The model under review builds one solid part; all positions refer to its coordinate system, in mm. Face numbers are marked on the shaded views. Give positions to 0.01 mm unless a question says otherwise; leave off trailing zeros. Loops run counter-clockwise (first coordinate to the right, second up) from the corner with the lowest first, then second, coordinate; pieces in that order, holes last. Notation, with made-up numbers: M -12.5,62.5 L 14.5,62.5 A21 ccw 14.5,96.5 Z; hole C 66.5,5.25 d4. An arc over 180 degrees is marked long. Return JSON: item names as keys, results as strings. Group by question number.
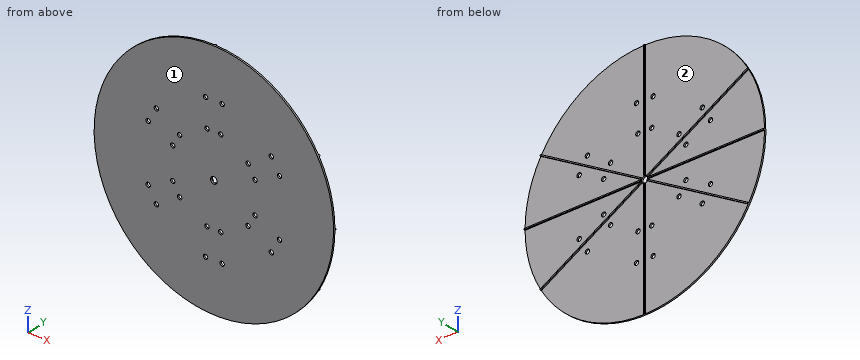
```python
from build123d import *

# Parameters (mm, degrees)
SKETCH1_R           = 217.5
SKETCH1_R_2         = 4
SKETCH1_R_3         = 6
BOSS_EXTRUDE1_DEPTH = 2.5
CUT_EXTRUDE1_START  = -2
SKETCH2_R           = 4
SKETCH2_R_2         = 6
CUT_EXTRUDE1_DEPTH  = 2


with BuildPart() as part:
    # Sketch1 → Boss-Extrude1 (new, symmetric)
    with BuildSketch(Plane(origin=(0, 0, 0), x_dir=(1, 0, 0), z_dir=(0, 1, 0))):
        with Locations(Location((0, 0, 0), (0, 0, 270))):
            Circle(SKETCH1_R)
        with Locations(Location((-12.5, 79.017403146, 0), (0, 0, 270))):
            Circle(SKETCH1_R_2, mode=Mode.SUBTRACT)
        with Locations(Location((12.5, 79.017403146, 0), (0, 0, 270))):
            Circle(SKETCH1_R_2, mode=Mode.SUBTRACT)
        with Locations(Location((62.181078466, 50.334019121, 0), (0, 0, 270))):
            Circle(SKETCH1_R_2, mode=Mode.SUBTRACT)
        with Locations(Location((74.681078466, 28.683384026, 0), (0, 0, 270))):
            Circle(SKETCH1_R_2, mode=Mode.SUBTRACT)
        with Locations(Location((74.681078466, -28.683384026, 0), (0, 0, 270))):
            Circle(SKETCH1_R_2, mode=Mode.SUBTRACT)
        with Locations(Location((62.181078466, -50.334019121, 0), (0, 0, 270))):
            Circle(SKETCH1_R_2, mode=Mode.SUBTRACT)
        with Locations(Location((12.5, -79.017403146, 0), (0, 0, 270))):
            Circle(SKETCH1_R_2, mode=Mode.SUBTRACT)
        with Locations(Location((-12.5, -79.017403146, 0), (0, 0, 270))):
            Circle(SKETCH1_R_2, mode=Mode.SUBTRACT)
        with Locations(Location((-62.181078466, -50.334019121, 0), (0, 0, 270))):
            Circle(SKETCH1_R_2, mode=Mode.SUBTRACT)
        with Locations(Location((-74.681078466, -28.683384026, 0), (0, 0, 270))):
            Circle(SKETCH1_R_2, mode=Mode.SUBTRACT)
        with Locations(Location((-74.681078466, 28.683384026, 0), (0, 0, 270))):
            Circle(SKETCH1_R_2, mode=Mode.SUBTRACT)
        with Locations(Location((-62.181078466, 50.334019121, 0), (0, 0, 270))):
            Circle(SKETCH1_R_2, mode=Mode.SUBTRACT)
        with Locations(Location((15, 129.131715701, 0), (0, 0, 270))):
            Circle(SKETCH1_R_2, mode=Mode.SUBTRACT)
        with Locations(Location((-15, 129.131715701, 0), (0, 0, 90))):
            Circle(SKETCH1_R_2, mode=Mode.SUBTRACT)
        with Locations(Location((104.331346232, 77.556238907, 0), (0, 0, 90))):
            Circle(SKETCH1_R_2, mode=Mode.SUBTRACT)
        with Locations(Location((119.331346232, 51.575476794, 0), (0, 0, 270))):
            Circle(SKETCH1_R_2, mode=Mode.SUBTRACT)
        with Locations(Location((119.331346232, -51.575476794, 0), (0, 0, 90))):
            Circle(SKETCH1_R_2, mode=Mode.SUBTRACT)
        with Locations(Location((104.331346232, -77.556238907, 0), (0, 0, 270))):
            Circle(SKETCH1_R_2, mode=Mode.SUBTRACT)
        with Locations(Location((15, -129.131715701, 0), (0, 0, 90))):
            Circle(SKETCH1_R_2, mode=Mode.SUBTRACT)
        with Locations(Location((-15, -129.131715701, 0), (0, 0, 270))):
            Circle(SKETCH1_R_2, mode=Mode.SUBTRACT)
        with Locations(Location((-104.331346232, -77.556238907, 0), (0, 0, 90))):
            Circle(SKETCH1_R_2, mode=Mode.SUBTRACT)
        with Locations(Location((-119.331346232, -51.575476794, 0), (0, 0, 270))):
            Circle(SKETCH1_R_2, mode=Mode.SUBTRACT)
        with Locations(Location((-119.331346232, 51.575476794, 0), (0, 0, 90))):
            Circle(SKETCH1_R_2, mode=Mode.SUBTRACT)
        with Locations(Location((-104.331346232, 77.556238907, 0), (0, 0, 270))):
            Circle(SKETCH1_R_2, mode=Mode.SUBTRACT)
        with Locations(Location((0, 0, 0), (0, 0, 270))):
            Circle(SKETCH1_R_3, mode=Mode.SUBTRACT)
    extrude(amount=BOSS_EXTRUDE1_DEPTH, both=True)

    # Sketch2 → Cut-Extrude1 (cut)
    with BuildSketch(Plane(origin=(0, 2.5, 0), x_dir=(1, 0, 0), z_dir=(0, 1, 0)).offset(CUT_EXTRUDE1_START)):
        with BuildLine():
            ThreePointArc((-217.497701137, -1), (-210.088867218, -56.29314231), (-188.85853445, -107.882825165))
            Line((-188.85853445, -107.882825165), (-5.888022785, -2.244751001))
            ThreePointArc((-5.888022785, -2.244751001), (-5.457177799, -3.150703071), (-4.888022785, -3.976801809))
            Line((-4.888022785, -3.976801809), (-187.85853445, -109.614875972))
            ThreePointArc((-187.85853445, -109.614875972), (-108.75, -188.360525323), (-1, -217.497701137))
            Line((-1, -217.497701137), (-1, -6.22155281))
            ThreePointArc((-1, -6.22155281), (0, -6.301406142), (1, -6.22155281))
            Line((1, -6.22155281), (1, -217.497701137))
            ThreePointArc((1, -217.497701137), (108.75, -188.360525323), (187.85853445, -109.614875972))
            Line((187.85853445, -109.614875972), (4.888022785, -3.976801809))
            ThreePointArc((4.888022785, -3.976801809), (5.457177799, -3.150703071), (5.888022785, -2.244751001))
            Line((5.888022785, -2.244751001), (188.85853445, -107.882825165))
            ThreePointArc((188.85853445, -107.882825165), (210.088867218, -56.29314231), (217.497701137, -1))
            Line((217.497701137, -1), (6.22155281, -1))
            ThreePointArc((6.22155281, -1), (6.301406142, 0), (6.22155281, 1))
            Line((6.22155281, 1), (217.497701137, 1))
            ThreePointArc((217.497701137, 1), (210.088867218, 56.29314231), (188.85853445, 107.882825165))
            Line((188.85853445, 107.882825165), (5.888022785, 2.244751001))
            ThreePointArc((5.888022785, 2.244751001), (5.457177799, 3.150703071), (4.888022785, 3.976801809))
            Line((4.888022785, 3.976801809), (187.85853445, 109.614875972))
            ThreePointArc((187.85853445, 109.614875972), (108.75, 188.360525323), (1, 217.497701137))
            Line((1, 217.497701137), (1, 6.22155281))
            ThreePointArc((1, 6.22155281), (0, 6.301406142), (-1, 6.22155281))
            Line((-1, 6.22155281), (-1, 217.497701137))
            ThreePointArc((-1, 217.497701137), (-108.75, 188.360525323), (-187.85853445, 109.614875972))
            Line((-187.85853445, 109.614875972), (-4.888022785, 3.976801809))
            ThreePointArc((-4.888022785, 3.976801809), (-5.457177799, 3.150703071), (-5.888022785, 2.244751001))
            Line((-5.888022785, 2.244751001), (-188.85853445, 107.882825165))
            ThreePointArc((-188.85853445, 107.882825165), (-210.088867218, 56.29314231), (-217.497701137, 1))
            Line((-217.497701137, 1), (-6.22155281, 1))
            ThreePointArc((-6.22155281, 1), (-6.301406142, 0), (-6.22155281, -1))
            Line((-6.22155281, -1), (-217.497701137, -1))
        make_face()
        with Locations(Location((-15, -129.131715701, 0), (0, 0, 270))):
            Circle(SKETCH2_R, mode=Mode.SUBTRACT)
        with Locations(Location((-119.331346232, -51.575476794, 0), (0, 0, 270))):
            Circle(SKETCH2_R, mode=Mode.SUBTRACT)
        with Locations(Location((-104.331346232, -77.556238907, 0), (0, 0, 90))):
            Circle(SKETCH2_R, mode=Mode.SUBTRACT)
        with Locations(Location((-12.5, -79.017403146, 0), (0, 0, 270))):
            Circle(SKETCH2_R, mode=Mode.SUBTRACT)
        with Locations(Location((-62.181078466, -50.334019121, 0), (0, 0, 270))):
            Circle(SKETCH2_R, mode=Mode.SUBTRACT)
        with Locations(Location((-74.681078466, -28.683384026, 0), (0, 0, 270))):
            Circle(SKETCH2_R, mode=Mode.SUBTRACT)
        with Locations(Location((15, -129.131715701, 0), (0, 0, 90))):
            Circle(SKETCH2_R, mode=Mode.SUBTRACT)
        with Locations(Location((12.5, -79.017403146, 0), (0, 0, 270))):
            Circle(SKETCH2_R, mode=Mode.SUBTRACT)
        with Locations(Location((104.331346232, -77.556238907, 0), (0, 0, 270))):
            Circle(SKETCH2_R, mode=Mode.SUBTRACT)
        with Locations(Location((62.181078466, -50.334019121, 0), (0, 0, 270))):
            Circle(SKETCH2_R, mode=Mode.SUBTRACT)
        with Locations(Location((74.681078466, -28.683384026, 0), (0, 0, 270))):
            Circle(SKETCH2_R, mode=Mode.SUBTRACT)
        with Locations(Location((119.331346232, -51.575476794, 0), (0, 0, 90))):
            Circle(SKETCH2_R, mode=Mode.SUBTRACT)
        with Locations(Location((-119.331346232, 51.575476794, 0), (0, 0, 90))):
            Circle(SKETCH2_R, mode=Mode.SUBTRACT)
        with Locations(Location((-74.681078466, 28.683384026, 0), (0, 0, 270))):
            Circle(SKETCH2_R, mode=Mode.SUBTRACT)
        with Locations(Location((-62.181078466, 50.334019121, 0), (0, 0, 270))):
            Circle(SKETCH2_R, mode=Mode.SUBTRACT)
        with Locations(Location((-104.331346232, 77.556238907, 0), (0, 0, 270))):
            Circle(SKETCH2_R, mode=Mode.SUBTRACT)
        with Locations(Location((-12.5, 79.017403146, 0), (0, 0, 270))):
            Circle(SKETCH2_R, mode=Mode.SUBTRACT)
        with Locations(Location((-15, 129.131715701, 0), (0, 0, 90))):
            Circle(SKETCH2_R, mode=Mode.SUBTRACT)
        with Locations(Location((0, 0, 0), (0, 0, 270))):
            Circle(SKETCH2_R_2, mode=Mode.SUBTRACT)
        with Locations(Location((74.681078466, 28.683384026, 0), (0, 0, 270))):
            Circle(SKETCH2_R, mode=Mode.SUBTRACT)
        with Locations(Location((62.181078466, 50.334019121, 0), (0, 0, 270))):
            Circle(SKETCH2_R, mode=Mode.SUBTRACT)
        with Locations(Location((12.5, 79.017403146, 0), (0, 0, 270))):
            Circle(SKETCH2_R, mode=Mode.SUBTRACT)
        with Locations(Location((104.331346232, 77.556238907, 0), (0, 0, 90))):
            Circle(SKETCH2_R, mode=Mode.SUBTRACT)
        with Locations(Location((119.331346232, 51.575476794, 0), (0, 0, 270))):
            Circle(SKETCH2_R, mode=Mode.SUBTRACT)
        with Locations(Location((15, 129.131715701, 0), (0, 0, 270))):
            Circle(SKETCH2_R, mode=Mode.SUBTRACT)
    extrude(amount=CUT_EXTRUDE1_DEPTH, mode=Mode.SUBTRACT)


solid = part.part
```
(1) Add section A-A (z = -142.5). Write out the cut boundary in (x, y).
(2) Add section B-B (y = -1.05). Count the separate pieces of the cut face and the enclosed holes in it, and give its area (3 significant figures).
(3) For probe 1 along X at (y, z) = (2.2, 32.5); probe 2 along X at (y, z) = (1.85, -19); probe 3 along Z at (x, y) = (29.5, 1.1), list the stretches that pass through material, from the lowest coordinate up.
(4) Add section D-D (z = 170.5). Write out the cut boundary in (x, y).
(5) Add section C-C (x = -180). Write out the cut boundary in (y, z).
(6) Mouldability with a two-part tool opening along X and no side actions: class the marked faces 1 and 2 as released by +X, released by -X, zero draft, split by the parting line, or undercut.
(7) For pin 1 (2 mm diameter, centred on y = 0, z = -164.5, fed in from +X); pin 2 (2 mm diameter, centred on x = -160, y = -0.5, fed in from +Z); pin 3 (5 mm diameter, centred on x = -74.68, z = -28.68, fed in from +Y); pin 4 (9 mm diameter, centred on x = -74.68, z = 28.68, fed in from +Y), all flat-tipped, find the tip position at first contact; note any pin that passes through.
Verdict:
{
 "1": {"outline": "M -164.32,-2.5 L 164.32,-2.5 L 164.32,0.5 L 1,0.5 L 1,2.5 L -1,2.5 L -1,0.5 L -164.32,0.5 Z"},
 "2": {"separate pieces": "1", "enclosed holes": "25", "area": "147,000 mm²"},
 "3": {"probe 1": "x = -58.29 to -54.29, -1 to 1, 54.29 to 58.29", "probe 2": "x = -34.91 to -30.91, -1 to 1, 30.91 to 34.91", "probe 3": "z = -18.19 to -15.88, -1 to 1, 15.88 to 18.19"},
 "4": {"outline": "M -135.04,-2.5 L 135.04,-2.5 L 135.04,0.5 L 1,0.5 L 1,2.5 L -1,2.5 L -1,0.5 L -135.04,0.5 Z"},
 "5": {"outline": "M -2.5,-122.09 L 0.5,-122.09 L 0.5,-105.08 L 2.5,-105.08 L 2.5,-102.77 L 0.5,-102.77 L 0.5,-1 L 2.5,-1 L 2.5,1 L 0.5,1 L 0.5,102.77 L 2.5,102.77 L 2.5,105.08 L 0.5,105.08 L 0.5,122.09 L -2.5,122.09 Z"},
 "6": {"face 1": "zero draft", "face 2": "undercut"},
 "7": {"pin 1": "stops at x = 143.44", "pin 2": "stops at z = 148.41", "pin 3": "passes through", "pin 4": "stops at y = 0.5"}
}
